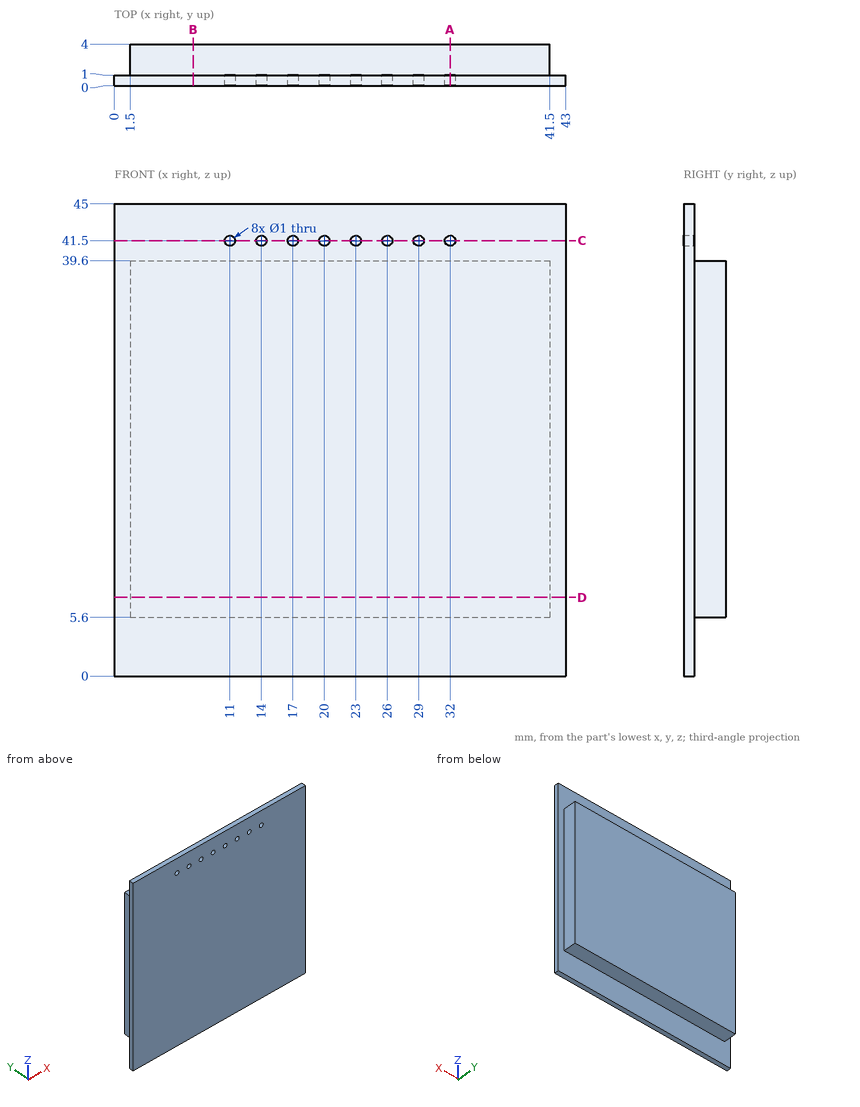
Can you work these out from the drawing? Everything is in mm from the part's minimum corner. Round coordinates to 2 decimals unless told otherwise and drop trailing zeros. Loops run counter-clockwise (first coordinate to the right, second up) from the corner with the lowest first, then second, coordinate; pieces in that order, holes last. Notation, with made-up numbers: (63, 40) - (102, 40) arc R21 ccw to (102, 59) - close; hole circle Ø11 at (69.25, -22). An arc over 180 degrees is marked (long way). Answer in a Markdown table with one row per item. Add a question column.
Q1. For pin 1 Ø0.9 at (x, y) = (15, 2.5) entering from +Z; pin 2 Ø0.9 at (x, y) = (24.5, 3) entering from -Z; pin 3 Ø0.9 at (y, z) = (3, 16.5) entering from -X, each with a flat end and sliding along its axis, tell me the tip position at first contact or that it passes through.
Q2. I want a section at A-A on x = 32. List the corners of the cut face in (y, z) for me, and give its area (3 significant figures).
Q3. I want a section at D-D on z = 7.5. List the corners of the cut face in (x, y) for me.
Q4. I want a section at C-C on z = 41.5. Count the separate pieces of the cut face and the enclosed holes in it, and give its area (3 significant figures).
Q5. I want a section at B-B on x = 7.5. List the corners of the cut face in (y, z) for me.
Q6. I need wall thicknesses on L1, parallel to Z at x = 23, y = 0.5; L2, parallel to Z at x = 26, y = 1.9; L3, parallel to X at y = 2.5, z = 18. Which ranges of each line are inside material? Lowest first, please.
A:
| question | item | result |
|---|---|---|
| 1 | pin 1 | z = 39.6 |
| 1 | pin 2 | z = 5.6 |
| 1 | pin 3 | x = 1.5 |
| 2 | outline | (0, 0) - (1, 0) - (1, 5.6) - (4, 5.6) - (4, 39.6) - (1, 39.6) - (1, 41) - (0, 41) - close; (0, 42) - (1, 42) - (1, 45) - (0, 45) - close |
| 2 | area | 146 mm^2 |
| 3 | outline | (0, 0) - (43, 0) - (43, 1) - (41.5, 1) - (41.5, 4) - (1.5, 4) - (1.5, 1) - (0, 1) - close |
| 4 | separate pieces | 9 |
| 4 | enclosed holes | 0 |
| 4 | area | 35.0 mm^2 |
| 5 | outline | (0, 0) - (1, 0) - (1, 5.6) - (4, 5.6) - (4, 39.6) - (1, 39.6) - (1, 45) - (0, 45) - close |
| 6 | L1 | 0 to 41, 42 to 45 |
| 6 | L2 | 5.6 to 39.6 |
| 6 | L3 | 1.5 to 41.5 |
